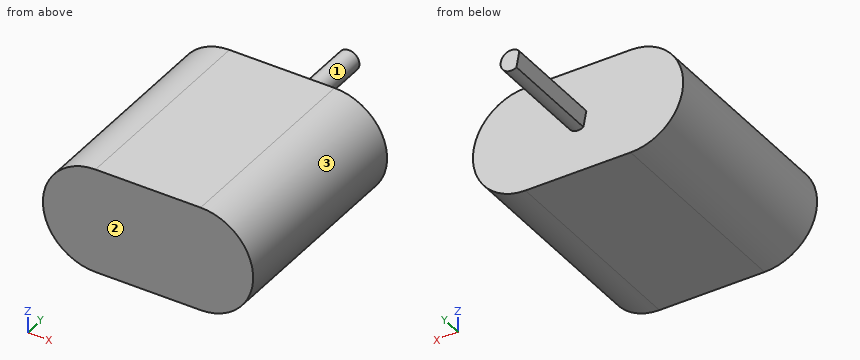
from build123d import *

# Parameters (mm, degrees)
BOSS_EXTRUDE1_DEPTH = 20
SKETCH4_R           = 1
BOSS_EXTRUDE2_DEPTH = 10
CUT_EXTRUDE1_START  = -10
CUT_EXTRUDE1_DEPTH  = 10


with BuildPart() as part:
    # Sketch1 → Boss-Extrude1 (new body)
    with BuildSketch(Plane(origin=(0, 0, 0), x_dir=(1, 0, 0), z_dir=(0, 1, 0))):
        with BuildLine():
            Line((0, 5), (10, 5))
            ThreePointArc((10, 5), (15, 0), (10, -5))
            Line((10, -5), (0, -5))
            ThreePointArc((0, -5), (-5, 0), (0, 5))
        make_face()
    extrude(amount=BOSS_EXTRUDE1_DEPTH)

    # Sketch4 → Boss-Extrude2 (add)
    with BuildSketch(Plane(origin=(0, 20, 0), x_dir=(1, 0, 0), z_dir=(0, 1, 0))):
        with Locations(Location((5, 0, 0), (0, 0, 270))):
            Circle(SKETCH4_R)
    extrude(amount=BOSS_EXTRUDE2_DEPTH)

    # Sketch5 → Cut-Extrude1 (cut)
    with BuildSketch(Plane(origin=(0, 30, 0), x_dir=(1, 0, 0), z_dir=(0, 1, 0)).offset(CUT_EXTRUDE1_START)):
        with BuildLine():
            Line((4.488521887, 0.859296305), (4.211378142, -0.614878497))
            ThreePointArc((4.211378142, -0.614878497), (4.017216799, 0.184762496), (4.488521887, 0.859296305))
        make_face()
    extrude(amount=CUT_EXTRUDE1_DEPTH, mode=Mode.SUBTRACT)


solid = part.part
Model file for the job. Use its own axes, mm. Face numbers are marked on the shaded views. Round coordinates to 2 decimals unless told otherwise and drop trailing zeros. Loops run counter-clockwise (first coordinate to the right, second up) from the corner with the lowest first, then second, coordinate; pieces in that order, holes last.
1. Band-saw the part on C-C, the plane z = 0. List the corners of the cut face in (x, y), and give its area (3 significant figures).
Check values:
outline: (-5, 0) - (15, 0) - (15, 20) - (6, 20) - (6, 30) - (4.33, 30) - (4.33, 20) - (-5, 20) - close
area: 417 mm2
2. Mould opens along X. For the marked faces 1, 2 and 3 say: +X half, -X half, draft (parallel to the pull), parting line (faces both ways), or undercut.
Check values:
face 1: parting line
face 2: draft
face 3: +X half
3. Band-saw the part on D-D, the plane y = 26. List the corners of the cut face in (x, z), and give its area (3 significant figures).
Check values:
outline: (4.21, 0.61) - (4.49, -0.86) arc R1 ccw (long way) to start
area: 2.79 mm2
4. Wall check: probe 1 along Y at (x, z) = (2.25, 1); probe 2 along X at (y, z) = (13.5, -4); probe 3 along X at (y, z) = (10, 2.75). Give the ranges that are in metal, low to high.
Check values:
probe 1: y = 0 to 20
probe 2: x = -3 to 13
probe 3: x = -4.18 to 14.18
5. Band-saw the part on B-B, the plane y = 15. List the corners of the cut face in (x, z), and give its area (3 significant figures).
Check values:
outline: (0, -5) - (10, -5) arc R5 ccw to (10, 5) - (0, 5) arc R5 ccw to start
area: 179 mm2
6. Drop flat-ended pins along their axis: P1, Ø1, axis at y = 15, z = -3, coming from the +X side; P2, Ø3, axis at x = 4.5, z = -2.5, coming from the +Y side; P3, Ø2, axis at y = 23, z = 0, coming from the +X side. Give the stop position or say it passes through.
Check values:
P1: stops at x = 14.33
P2: stops at y = 20
P3: stops at x = 6
7. Band-saw the part on A-A, the plane x = 5. List the corners of the cut face in (y, z).
Check values:
outline: (0, -5) - (20, -5) - (20, -1) - (30, -1) - (30, 1) - (20, 1) - (20, 5) - (0, 5) - close
